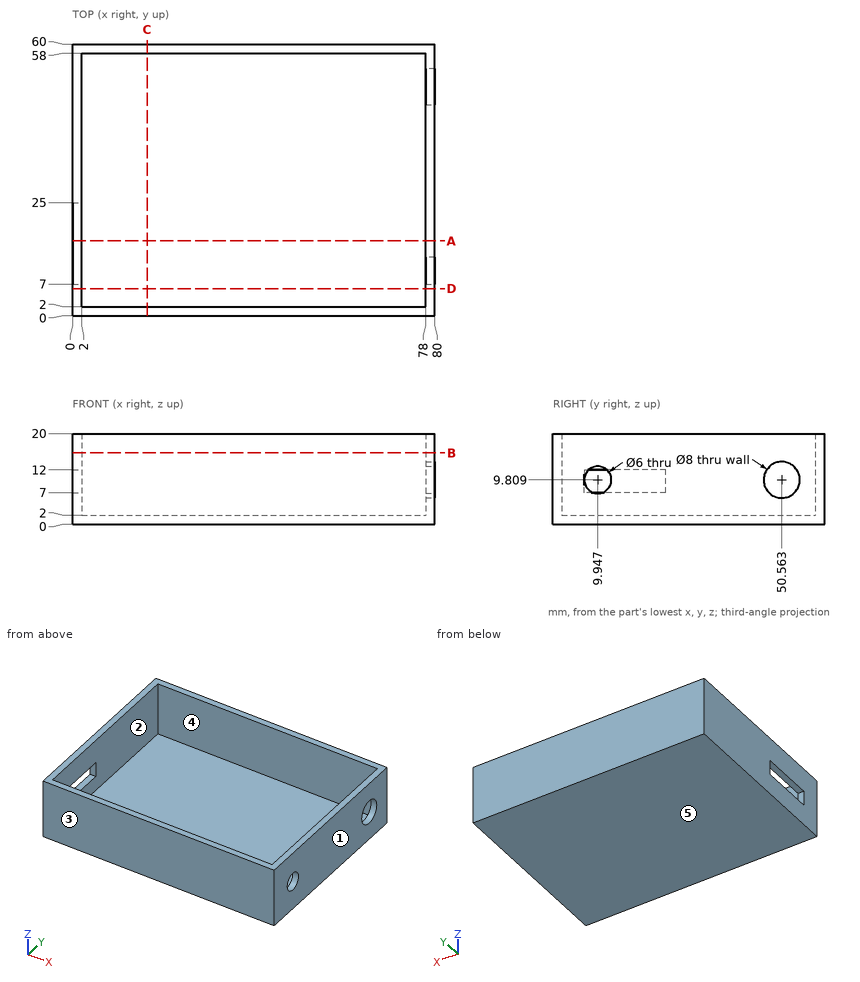
Here's the drawing with two shaded views (mm, measured from the low corner). I have some questions. A direction names the side the tool comes from. Coordinates: 2 decimals unless noted, no trailing zeros. Write each loop counter-clockwise with the first axis right and the second up, starting at its lowest first coordinate (ties: lowest second). Pieces come first, ordered by that corner, then holes. Notation, with made-up numbers: M 57,-34.5 L 73,-34.5 A34 cw 73,1.5 Z; hole C 21.5,57.5 d2. An arc over 180 degrees is marked long. Write item = value, one per line. Start each with the question number.
Q1. If we section it at C-C, the plane x = 16.5: Write out the boundary of the cut face in (y, z).
Q2. Thinking about a two-plate mould opening in Y: for the marked faces 3, 4 and 5, which applies, released by +Y, released by -Y, zero draft, split by the parting line, or undercut?
Q3. If we section it at B-B, the plane z = 15.75: Write out the boundary of the cut face in (x, y).
Q4. If we section it at D-D, the plane y = 6: Write out the boundary of the cut face in (x, z).
Q5. On a 3-axis mill with a long thin cutter (end or side, diameter ignored), from which of +Z, -Z, +X, -X, +Y, -Y can I reach the whole of each face in a straight line? I mean the marked faces 1 and 2. Say none if no direction works.
Q6. I'm going to push flat-ended pins straight in: pin 1 (17 mm diameter, centred on x = 48, y = 43, fed in from +Z); pin 2 (6.5 mm diameter, centred on y = 50.56, z = 9.81, fed in from +X). Where does each tip first touch, or does it pass through?
Q7. If I drill on L1, parallel to Y at x = 16, z = 13.5; L2, parallel to X at y = 27.5, z = 6.75; L3, parallel to Z at x = 23.5, y = 52, over which ranges is the centre line in solid material (lowest first)? Write a range as [from, to].
Q8. If we section it at A-A, the plane y = 16.5: Write out the boundary of the cut face in (x, z), then the cut area to 3 significant figures.
Check sheet entries:
q1.outline = M 0,0 L 60,0 L 60,20 L 58,20 L 58,2 L 2,2 L 2,20 L 0,20 Z
q2.face_3 = released by -Y
q2.face_4 = undercut
q2.face_5 = zero draft
q3.outline = M 0,0 L 80,0 L 80,60 L 0,60 Z; hole M 2,2 L 78,2 L 78,58 L 2,58 Z
q4.outline = M 0,0 L 80,0 L 80,20 L 78,20 L 78,2 L 2,2 L 2,20 L 0,20 Z
q5.face_1 = +Z, -Z, +X, +Y, -Y
q5.face_2 = +Z
q6.pin_1 = 2
q6.pin_2 = 2
q7.L1 = [0, 2], [58, 60]
q7.L2 = [0, 2], [78, 80]
q7.L3 = [0, 2]
q8.outline = M 0,0 L 80,0 L 80,20 L 78,20 L 78,2 L 2,2 L 2,7 L 0,7 Z; M 0,12 L 2,12 L 2,20 L 0,20 Z
q8.area = 222 mm²
